Part print with two shaded views. Sizes in mm from the minimum x, y, z corner. A direction names the side the tool comes from. Give positions to 0.01 mm unless a question says otherwise; leave off trailing zeros. Write each loop counter-clockwise with the first axis right and the second up, starting at its lowest first coordinate (ties: lowest second). Pieces come first, ordered by that corner, then holes. Notation, with made-up numbers: (-35, -8) -> (1, -8) arc R25 cw to (1, 22) -> close; hole circle Ø1 at (-4.5, -17). An arc over 180 degrees is marked (long way). Answer in a Markdown table with one row per item. Add a question column.
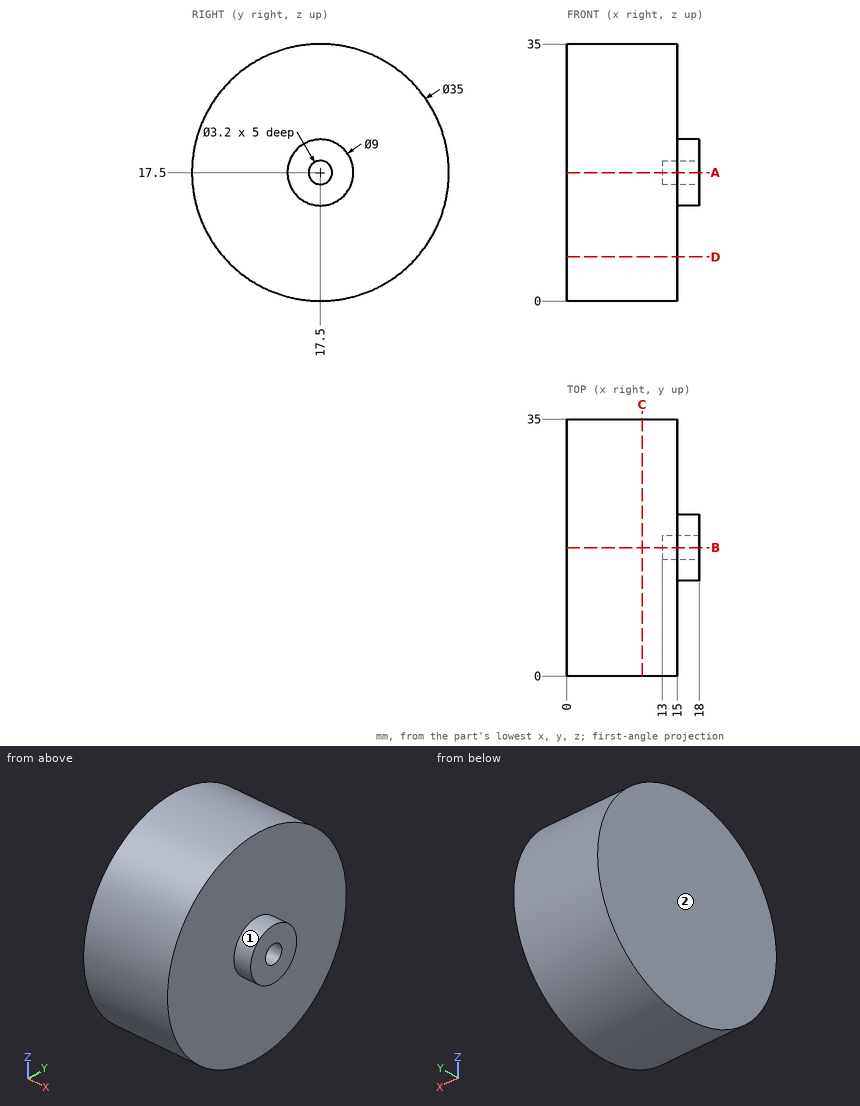
Item 1: Slice it at D-D, the plane z = 6. List the corners of the cut face in (x, y), then the cut area to 3 significant figures.
Item 2: Drop flat-ended pins along their axis: pin 1 Ø5 at (x, y) = (13.5, 10) entering from -Z; pin 2 Ø10 at (x, y) = (3, 10.5) entering from +Z; pin 3 Ø4 at (x, y) = (5.5, 7.5) entering from +Z. Give the stop position or say it passes through.
Item 3: Probe L1, parallel to Z at x = 15.4, y = 17.5; L2, parallel to Z at x = 14.4, y = 17.5; L3, parallel to X at y = 10, z = 21.5. List the from-to ranges inside material, lowest first. Write a range as from..to.
Item 4: Slice it at A-A, the plane z = 17.5. List the corners of the cut face in (x, y), then the cut area to 3 significant figures.
Item 5: Which spindle directions (+Z, -Z, +X, -X, +Y, -Y) get a long thin tool onto all of the face, cutting with end or side? Do the marked faces 1 and 2. Say none if no direction does.
Item 6: Slice it at C-C, the plane x = 10.25. List the corners of the cut face in (y, z), then the cut area to 3 significant figures.
Answer key:
| question | item | result |
|---|---|---|
| 1 | outline | (0, 4.31) -> (15, 4.31) -> (15, 30.69) -> (0, 30.69) -> close |
| 1 | area | 396 mm² |
| 2 | pin 1 | stops at z = 0.73 |
| 2 | pin 2 | stops at z = 34.89 |
| 2 | pin 3 | stops at z = 33.06 |
| 3 | L1 | z = 13..15.9, 19.1..22 |
| 3 | L2 | z = 0..15.9, 19.1..35 |
| 3 | L3 | x = 0..15 |
| 4 | outline | (0, 0) -> (15, 0) -> (15, 13) -> (18, 13) -> (18, 15.9) -> (13, 15.9) -> (13, 19.1) -> (18, 19.1) -> (18, 22) -> (15, 22) -> (15, 35) -> (0, 35) -> close |
| 4 | area | 536 mm² |
| 5 | face 1 | +X |
| 5 | face 2 | +Z, -Z, -X, +Y, -Y |
| 6 | outline | circle Ø35 at (17.5, 17.5) |
| 6 | area | 962 mm² |
